from build123d import *

# Parameters (mm, degrees)
F1_DEPTH = 10
F3_D     = 4


with BuildPart() as f1:
    # F0 (on Top) → F1 (new body)
    with BuildSketch(Plane.XY):
        Polygon((-2.086833, -10.936922), (10.913167, -10.936922), (10.913167, -7.936922), (0.913167, -7.936922), (0.913167, 9.063078), (-9.498044, 9.063078), (-13.724226, 0), (-10.414093, 0), (-7.586833, 6.063078), (-2.086833, 6.063078), align=None)
    extrude(amount=F1_DEPTH)

    # F3 (through all)
    with Locations(Plane(origin=(0, -7.936922, 0), x_dir=(-1, 0, 0), z_dir=(0, 1, 0))):
        with Locations((-5.913167, 5)):
            Hole(F3_D / 2)


solid = f1.part
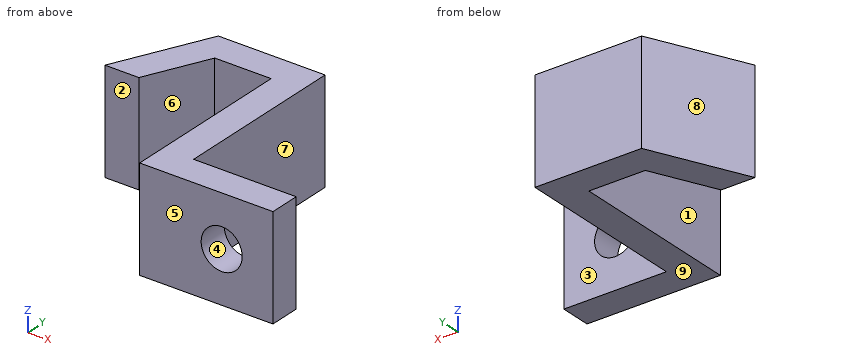
CAD build for the part. Positions are in the model's coordinates, mm. Face numbers are marked on the shaded views. A direction names the side the tool comes from. Round coordinates to 2 decimals unless told otherwise and drop trailing zeros. Loops run counter-clockwise (first coordinate to the right, second up) from the corner with the lowest first, then second, coordinate; pieces in that order, holes last.
(1) Wall check: line 1 along X through (y, z) = (-4.5, 2.75); line 2 along Y through (x, z) = (-6.75, 0.75); line 3 along X through (y, z) = (3.75, 8). Give the ranges that are in metal, low to high.
(2) Cut at C-C (y = 1.5). Give the cut face in (x, z), plus the area to 3 significant figures.
(3) Cut at B-B (x = 5.5). Give the cut face in (y, z).
(4) Which spindle directions (+Z, -Z, +X, -X, +Y, -Y) get a long thin tool onto all of the face, cutting with end or side? Do the marked faces 1, 2, 3, 4 and 5. Say none if no direction does.
(5) Drop flat-ended pins along their axis: pin 1 (3 mm diameter, centred on y = -3, z = 4.5, fed in from -X); pin 2 (1.5 mm diameter, centred on x = 7.5, z = 6, fed in from +Y); pin 3 (3 mm diameter, centred on x = -4, z = 3, fed in from -Y). Give the stop position or say it passes through.
(6) Cut at A-A (z = 5). Give the cut face in (x, y), plus the area to 3 significant figures.
(7) Cut at D-D (z = 9). Give the cut face in (x, y), plus the area to 3 significant figures.
(8) Two-plate mould, pull along X, no slides. Class the marked faces 6, 7, 8 and 9: +X half, -X half, draft (parallel to the pull), parting line (faces both ways), or undercut.
Findings below:
1. line 1: x = -2.09 to 0.91
1. line 2: y = 6.06 to 9.06
1. line 3: x = -11.98 to -8.67, -2.09 to 0.91
2. outline: (-13.02, 0) - (-9.71, 0) - (-9.71, 10) - (-13.02, 10) - close; (-2.09, 0) - (0.91, 0) - (0.91, 10) - (-2.09, 10) - close
2. area: 63.1 mm2
3. outline: (-10.94, 0) - (-7.94, 0) - (-7.94, 3.04) - (-10.94, 3.04) - close; (-10.94, 6.96) - (-7.94, 6.96) - (-7.94, 10) - (-10.94, 10) - close
4. face 1: +Z, -Z, -Y
4. face 2: +Z, -Z, -X, -Y
4. face 3: +Z, -Z, +X, +Y
4. face 4: +Y, -Y
4. face 5: +Z, -Z, +X, -X, -Y
5. pin 1: stops at x = -2.09
5. pin 2: stops at y = -7.94
5. pin 3: stops at y = 6.06
6. outline: (-13.72, 0) - (-10.41, 0) - (-7.59, 6.06) - (-2.09, 6.06) - (-2.09, -10.94) - (3.91, -10.94) - (3.91, -7.94) - (0.91, -7.94) - (0.91, 9.06) - (-9.5, 9.06) - close; (7.91, -10.94) - (10.91, -10.94) - (10.91, -7.94) - (7.91, -7.94) - close
6. area: 122 mm2
7. outline: (-13.72, 0) - (-10.41, 0) - (-7.59, 6.06) - (-2.09, 6.06) - (-2.09, -10.94) - (10.91, -10.94) - (10.91, -7.94) - (0.91, -7.94) - (0.91, 9.06) - (-9.5, 9.06) - close
7. area: 134 mm2
8. face 6: undercut
8. face 7: +X half
8. face 8: -X half
8. face 9: draft
